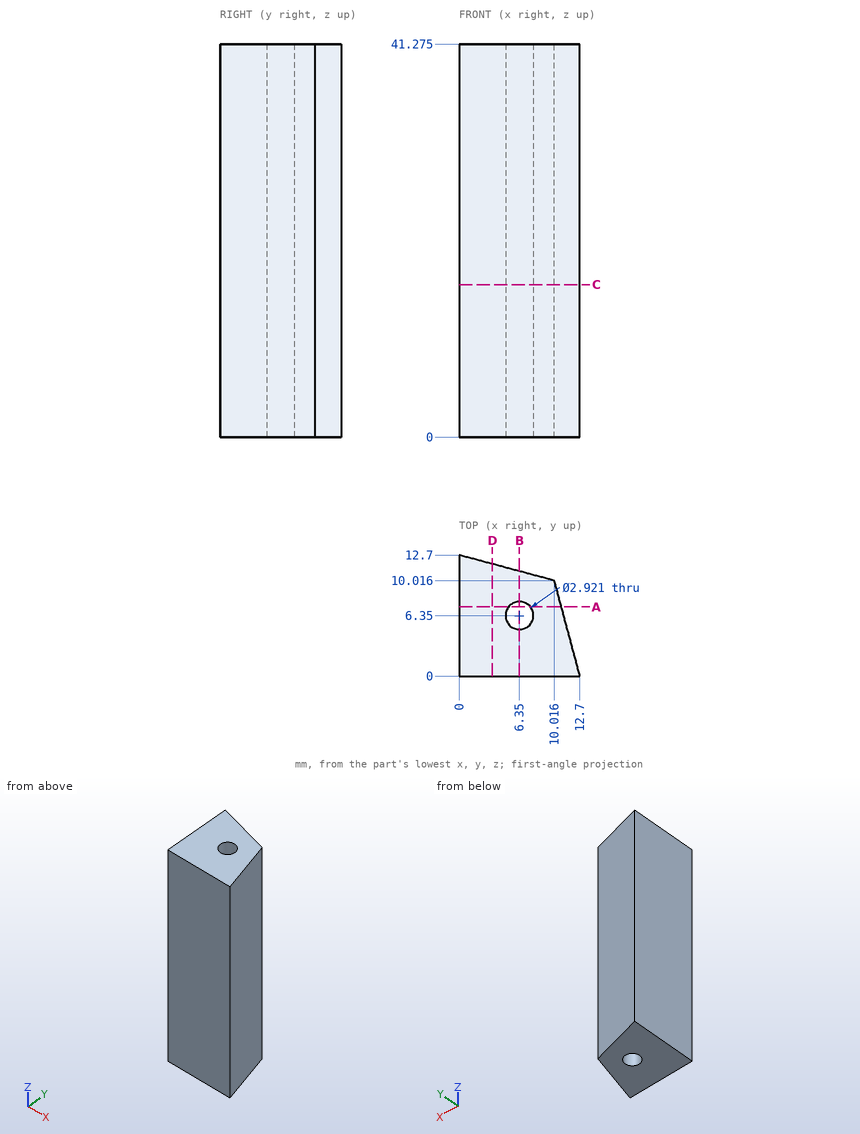
Job drawing, mm, ordinate dimensions from the low corner. One solid piece. Coordinates: 2 decimals unless noted, no trailing zeros. Order: outer loops, then holes, each group sorted by start corner. A loop starts at its lowest first (then second) coordinate and runs counter-clockwise, first axis right, second up. Notation, with made-up numbers: (22, -10) -> (35, -10) arc R31 cw to (35, 22) -> close; hole circle Ø8 at (20, 46). An arc over 180 degrees is marked (long way). Answer in a Markdown table with one row per item. Add a question column.
Q1. Band-saw the part on A-A, the plane y = 7.25. List the corners of the cut face in (x, z) (1 decimal).
Q2. Wall check: line 1 along Y through (x, z) = (6.35, 26.5); line 2 along Y through (x, z) = (5.25, 38); line 3 along Y through (x, z) = (1.5, 25.5). Give the ranges that are in metal, low to high. Write a range as [from, to].
Q3. Drop flat-ended pins along their axis: pin 1 (1.5 mm diameter, centred on x = 4.5, y = 10.5, fed in from -Z); pin 2 (4 mm diameter, centred on x = 6, z = 33.5, fed in from +Y); pin 3 (2.5 mm diameter, centred on x = 6.35, y = 6.35, fed in from -Z). Give the stop position or say it passes through.
Q4. Band-saw the part on D-D, the plane x = 3.5. List the corners of the cut face in (y, z) (1 decimal).
Q5. Band-saw the part on C-C, the plane z = 16. List the corners of the cut face in (x, y).
Q6. Band-saw the part on B-B, the plane x = 6.35. List the corners of the cut face in (y, z) (1 decimal).
Answers follow:
| question | item | result |
|---|---|---|
| 1 | outline | (0, 0) -> (5.2, 0) -> (5.2, 41.3) -> (0, 41.3) -> close; (7.5, 0) -> (10.8, 0) -> (10.8, 41.3) -> (7.5, 41.3) -> close |
| 2 | line 1 | [0, 4.89], [7.81, 11] |
| 2 | line 2 | [0, 5.39], [7.31, 11.29] |
| 2 | line 3 | [0, 12.3] |
| 3 | pin 1 | z = 0 |
| 3 | pin 2 | y = 11.63 |
| 3 | pin 3 | through |
| 4 | outline | (0, 0) -> (11.8, 0) -> (11.8, 41.3) -> (0, 41.3) -> close |
| 5 | outline | (0, 0) -> (12.7, 0) -> (10.02, 10.02) -> (0, 12.7) -> close; hole circle Ø2.92 at (6.35, 6.35) |
| 6 | outline | (0, 0) -> (4.9, 0) -> (4.9, 41.3) -> (0, 41.3) -> close; (7.8, 0) -> (11, 0) -> (11, 41.3) -> (7.8, 41.3) -> close |
